Could you check a few things on this model? Use its own coordinates, in mm. A direction names the side the tool comes from. Coordinates: 2 decimals unless noted, no trailing zeros. Loops run counter-clockwise (first coordinate to the right, second up) from the corner with the lowest first, then second, coordinate; pieces in that order, holes last.
1) Will these pins go through, and if not, where does the flat tip stop? P1, Ø2, axis at y = -6.5, z = -0.5, coming from the +X side; P2, Ø12, axis at x = 178, z = 0.5, coming from the -Y side; P3, Ø20, axis at x = 177, z = 6.5, coming from the +Y side; P4, Ø1.9, axis at x = -21, z = 0, coming from the +Y side.
2) Imagine slicing it at D-D on x = 98. Please give me the cut outline in (y, z).
3) Imagine slicing it at B-B on x = -7. Please give me the cut outline in (y, z), plus the area to 3 significant figures.
4) Imagine slicing it at C-C on z = 13.5. Please give me the cut outline in (x, y), plus the area to 3 significant figures.
5) Thinking about a two-plate mould opening in X: for faces 5 (the face through (143, 9, 0)), 6 (the face through (132, -4, 6)), 7 (the face through (-25, 0, 0)), which applies, released by +X, released by -X, zero draft, split by the parting line, or undercut?
6) For faces 1 (the face through (143, -9, 0)), 2 (the face through (-12, 0, 9.5)), 3 (the face through (247.99, -0.07, -0.62)), 4 (the face through (0, -7, -2)), which set-ups out of +Z, -Z, +X, -X, +Y, -Y let a thin tool reach every point of the face, with its end or its side?
7) If I drill on line 1 along Z through (x, y) = (-21, 2.25); line 2 along Y through (x, z) = (155.5, 0); line 3 along X through (y, z) = (-5.5, -1), over which ranges is the centre line in solid material (lowest first)?
8) Imagine slicing it at A-A on y = 0. Please give me the cut outline in (x, z).
```python
from build123d import *

# Parameters (mm, degrees)
F0_W     = 132
F0_H     = 7
F2_DEPTH = 9
F3_DEPTH = 5
F0_R     = 1.55
F4_DEPTH = 10


with BuildPart() as f1:
    # F0 (on Front) → F1 (revolve)
    with BuildSketch(Plane.XZ):
        with Locations((66, -3.5)):
            Rectangle(F0_W, F0_H)
    revolve(axis=Axis((66, 0, 0), (1, 0, 0)))

    # F0 (on Front) → F2 (join, symmetric)
    with BuildSketch(Plane.XZ):
        Polygon((132, 9), (132, 0), (132, -7), (132, -9), (151, -9), (154, -9), (154, 9), (151, 9), align=None)
    extrude(amount=F2_DEPTH, both=True)

    # F0 (on Front) → F3 (join, symmetric)
    with BuildSketch(Plane.XZ):
        with BuildLine():
            Line((160, 18), (151, 9))
            Line((151, 9), (154, 9))
            Line((154, 9), (154, -9))
            Line((154, -9), (151, -9))
            Line((151, -9), (160, -18))
            Line((160, -18), (216, -16))
            ThreePointArc((216, -16), (248, 0), (216, 16))
            Line((216, 16), (160, 18))
        make_face()
    extrude(amount=F3_DEPTH, both=True)

    # F0 (on Front) → F4 (join, symmetric)
    with BuildSketch(Plane.XZ):
        Polygon((0, -7), (0, 0), (0, 9.5), (-25, 9.5), (-25, -9.5), (0, -9.5), align=None)
        with Locations((-21, 0)):
            Circle(F0_R, mode=Mode.SUBTRACT)
    extrude(amount=F4_DEPTH, both=True)


solid = f1.part
```
Filled in:
1. P1: stops at x = 154
1. P2: stops at y = -5
1. P3: stops at y = 5
1. P4: passes through
2. outline: circle Ø14 at (0, 0)
3. outline: (-10, -9.5) - (10, -9.5) - (10, 9.5) - (-10, 9.5) - close
3. area: 380 mm2
4. outline: (155.5, -5) - (242.76, -5) - (242.76, 5) - (155.5, 5) - close
4. area: 873 mm2
5. face 5: zero draft
5. face 6: undercut
5. face 7: released by -X
6. face 1: +Z, -Z, +X, -Y
6. face 2: +Z, -X, +Y, -Y
6. face 3: +Y, -Y
6. face 4: none
7. line 1: z = -9.5 to -1.55, 1.55 to 9.5
7. line 2: y = -5 to 5
7. line 3: x = -25 to -22.18, -19.82 to 154
8. outline: (-25, -9.5) - (0, -9.5) - (0, -7) - (132, -7) - (132, -9) - (151, -9) - (160, -18) - (216, -16) arc R20 ccw (long way) to (216, 16) - (160, 18) - (151, 9) - (132, 9) - (132, 7) - (0, 7) - (0, 9.5) - (-25, 9.5) - close; hole circle Ø3.1 at (-21, 0)
